The model under review builds one solid part; all positions refer to its coordinate system, in mm. Face numbers are marked on the shaded views. A direction names the side the tool comes from. Round coordinates to 2 decimals unless told otherwise and drop trailing zeros. Write each loop counter-clockwise with the first axis right and the second up, starting at its lowest first coordinate (ties: lowest second). Pieces come first, ordered by that corner, then holes. Notation, with made-up numbers: (23, 64) - (46, 64) arc R27 ccw to (46, 97) - close; hole circle Ø7 at (-14, -2). An arc over 180 degrees is marked (long way). Return JSON: item names as keys, results as strings.
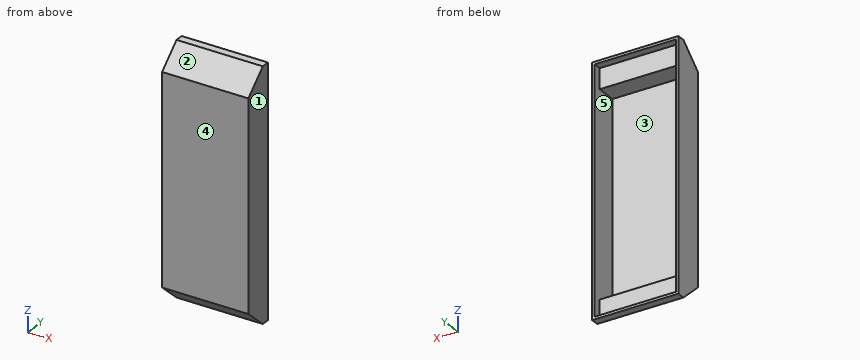
from build123d import *

# Parameters (mm, degrees)
BOSS_EXTRUDE1_DEPTH = 26.9875
BOSS_EXTRUDE2_DEPTH = 1.5875


with BuildPart() as part:
    # Sketch3 → Boss-Extrude1 (new, symmetric)
    with BuildSketch(Plane(origin=(0, 0, 0), x_dir=(0, 0, -1), z_dir=(1, 0, 0))):
        Polygon((95.5744504, 32.516625584), (108.2744504, 46.804125584), (108.2744504, 51.804125584), (106.6869504, 51.804125584), (106.6869504, 46.804125584), (93.9869504, 46.804125584), (93.9869504, 34.104125584), (-33.0130496, 34.104125584), (-33.0130496, 46.804125584), (-45.7130496, 46.804125584), (-45.7130496, 51.804125584), (-47.3005496, 51.804125584), (-47.3005496, 46.804125584), (-34.6005496, 32.516625584), align=None)
    extrude(amount=BOSS_EXTRUDE1_DEPTH, both=True)

    # Sketch4 → Boss-Extrude2 (add)
    with BuildSketch(Plane(origin=(26.9875, 0, 0), x_dir=(0, 0, -1), z_dir=(1, 0, 0))):
        Polygon((-33.0130496, 46.804125584), (-33.0130496, 34.104125584), (93.9869504, 34.104125584), (93.9869504, 46.804125584), (108.2744504, 46.804125584), (108.2744504, 51.804125584), (-47.3005496, 51.804125584), (-47.3005496, 46.804125584), align=None)
    boss_extrude2 = extrude(amount=-BOSS_EXTRUDE2_DEPTH)

    # Mirror1: Boss-Extrude2 across plane
    add(boss_extrude2.mirror(Plane(origin=(0, 0, 0), x_dir=(0, 0, 1), z_dir=(1, 0, 0))))


solid = part.part
(1) Wall thickness on line 1 (X direction, y = 44, z = -8); line 2 (Z direction, x = -10.5, y = 48.25); line 3 (Y direction, x = 24, z = -22): over which ranges is each line inside the solid? List them lowest first.
Filled in:
{"line 1": "x = -26.99 to -25.4, 25.4 to 26.99", "line 2": "z = -108.27 to -106.69, 45.71 to 47.3", "line 3": "y = 32.52 to 34.1"}
(2) For the marked faces 4 and 5, list the 3-axis set-ups (+Z, -Z, +X, -X, +Y, -Y) from which the entire face can be reached by the end or side of a thin tool; tool diameter is ignored.
Filled in:
{"face 4": "+Z, -Z, +X, -X, -Y", "face 5": "+Y"}
(3) Add section B-B (x = 7). Write out the cut boundary in (y, z), plus the area to 3 significant figures.
Filled in:
{"outline": "(32.52, -95.57) - (46.8, -108.27) - (51.8, -108.27) - (51.8, -106.69) - (46.8, -106.69) - (46.8, -93.99) - (34.1, -93.99) - (34.1, 33.01) - (46.8, 33.01) - (46.8, 45.71) - (51.8, 45.71) - (51.8, 47.3) - (46.8, 47.3) - (32.52, 34.6) - close", "area": "444 mm2"}
(4) Mouldability with a two-part tool opening along Z and no side actions: class the marked faces 1, 2 and 3 as released by +Z, released by -Z, zero draft, split by the parting line, or undercut.
Filled in:
{"face 1": "zero draft", "face 2": "released by +Z", "face 3": "undercut"}
(5) Add section A-A (y = 49.25). Write out the cut boundary in (x, z), plus the area to 3 significant figures.
Filled in:
{"outline": "(-26.99, -108.27) - (26.99, -108.27) - (26.99, 47.3) - (-26.99, 47.3) - close; hole (-25.4, -106.69) - (25.4, -106.69) - (25.4, 45.71) - (-25.4, 45.71) - close", "area": "655 mm2"}
(6) Clearance check with flat-ended pins moving along their axes: pin 1 Ø4 at (x, y) = (-8, 42.5) entering from +Z; pin 2 Ø6 at (x, z) = (-10, -86.5) entering from +Y; pin 3 Ø10 at (x, z) = (0.5, 40.5) entering from +Y. State where each tip first meets the part, or that it passes through.
Filled in:
{"pin 1": "stops at z = 45.25", "pin 2": "stops at y = 34.1", "pin 3": "stops at y = 46.8"}
(7) Add section C-C (z = -82.5). Write out the cut boundary in (x, y).
Filled in:
{"outline": "(-26.99, 32.52) - (26.99, 32.52) - (26.99, 51.8) - (25.4, 51.8) - (25.4, 34.1) - (-25.4, 34.1) - (-25.4, 51.8) - (-26.99, 51.8) - close"}
(8) Add section D-D (y = 38). Write out the cut boundary in (x, z), plus the area to 3 significant figures.
Filled in:
{"outline": "(-26.99, -100.45) - (26.99, -100.45) - (26.99, 39.47) - (-26.99, 39.47) - close; hole (-25.4, -93.99) - (25.4, -93.99) - (25.4, 33.01) - (-25.4, 33.01) - close", "area": "1,100 mm2"}
